Here's the drawing with two shaded views (mm, measured from the low corner). I have some questions. A direction names the side the tool comes from. Round coordinates to 2 decimals unless told otherwise and drop trailing zeros. Loops run counter-clockwise (first coordinate to the right, second up) from the corner with the lowest first, then second, coordinate; pieces in that order, holes last. Notation, with made-up numbers: M 76.25,-13.5 L 97.25,-13.5 A17 ccw 97.25,-1.5 Z; hole C -34,67 d5. An arc over 180 degrees is marked long. Answer as CSV lines item,"result".
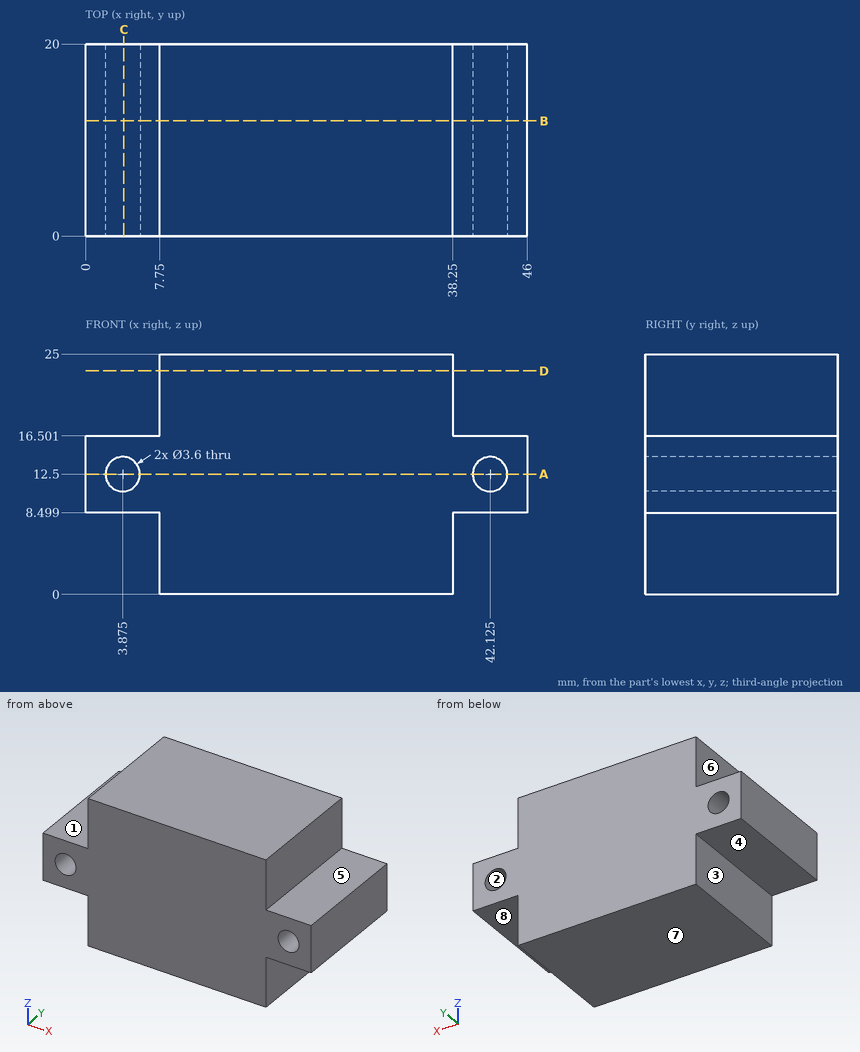
1. We'd pull the mould along X, two halves only. Please class the marked faces 1, 2 and 3: pulls with the +X half, pulls with the -X half, needs draft (parallel to the pull), parting line crosses it, or undercut.
Evaluation:
face 1,"needs draft"
face 2,"undercut"
face 3,"pulls with the -X half"
2. Which directions (+Z, -Z, +X, -X, +Y, -Y) give clear straight access to the entire face, cutting with the end or side of a thin tool? Please do the marked faces 4, 5, 6, 7 and 8.
Evaluation:
face 4,"-Z, -X, +Y, -Y"
face 5,"+Z, +X, +Y, -Y"
face 6,"+Z, -X, +Y, -Y"
face 7,"-Z, +X, -X, +Y, -Y"
face 8,"-Z, +X, +Y, -Y"
3. I want a section at A-A, the plane z = 12.5. Please give me the cut outline in (x, y) (1 decimal), and give its area (3 significant figures).
Evaluation:
outline,"M 0,0 L 2.1,0 L 2.1,20 L 0,20 Z; M 5.7,0 L 40.3,0 L 40.3,20 L 5.7,20 Z; M 43.9,0 L 46,0 L 46,20 L 43.9,20 Z"
area,"776 mm²"
4. If I drill on line 1 (X direction, y = 11.75, z = 12.5) (1 decimal); line 2 (X direction, y = 5.5, z = 2.25); line 3 (Z direction, x = 44, y = 6.25), over which ranges is the centre line in solid material (lowest first)? Write a range as [from, to].
Evaluation:
line 1,"x = [0, 2.1], [5.7, 40.3], [43.9, 46]"
line 2,"x = [7.75, 38.25]"
line 3,"z = [8.5, 16.5]"
5. I want a section at B-B, the plane y = 12. Count the separate pieces of the cut face and the enclosed holes in it, and give its area (3 significant figures).
Evaluation:
separate pieces,"1"
enclosed holes,"2"
area,"866 mm²"
6. I want a section at C-C, the plane x = 4. Please give me the cut outline in (y, z) (1 decimal).
Evaluation:
outline,"M 0,8.5 L 20,8.5 L 20,10.7 L 0,10.7 Z; M 0,14.3 L 20,14.3 L 20,16.5 L 0,16.5 Z"
7. I want a section at D-D, the plane z = 23.25. Please give me the cut outline in (x, y), and give its area (3 significant figures).
Evaluation:
outline,"M 7.75,0 L 38.25,0 L 38.25,20 L 7.75,20 Z"
area,"610 mm²"
8. For P1, Ø2.5, axis at y = 9, z = 19, coming from the -X side; P2, Ø4, axis at x = 3, y = 9, coming from the +Z side; P3, Ø2.5, axis at x = 43.5, y = 12, coming from the -Z side, each with a flat end and sliding along its axis, tell me the tip position at first contact or that it passes through.
Evaluation:
P1,"stops at x = 7.75"
P2,"stops at z = 16.5"
P3,"stops at z = 8.5"
